Verification items for the finished model (mm, model axes). A direction names the side the tool comes from. Round coordinates to 2 decimals unless told otherwise and drop trailing zeros. Write each loop counter-clockwise with the first axis right and the second up, starting at its lowest first coordinate (ties: lowest second). Pieces come first, ordered by that corner, then holes. Notation, with made-up numbers: (-1, -39.75) - (21, -39.75) arc R22 ccw to (21, -29.75) - close; hole circle Ø7 at (-28, 8.5). An arc over 180 degrees is marked (long way). Answer as a JSON object with one key per item and string values. Group by question number.
1) Mould release check, pull along Z, two halves, no side actions. Record for faces 4 (the cylindrical face through (105.83, 3.42, 37.39)), 5 (the cylindrical face through (6.1, 8.35, 33.76)), 6 (the cylindrical face through (5.92, 3.42, -37.39)), 7 (the flat face through (0, 18, -1)): +Z half, -Z half, draft (parallel to the pull), parting line (faces both ways), or undercut.
2) Section check D-D (z = 26). State how many separate pieces and enclosed holes the cut face has, then the cut area to 3 significant figures.
3) Section check B-B (z = -16.5). Enter the section's corners in (x, y), then the cut area to 3 significant figures.
4) Set-up check for faces 1 (the flat face through (94, 53, 23)), 2 (the flat face through (69, 46, -6)), 3 (the flat face through (54, 24, -1)): record each of +Z, -Z, +X, -X, +Y, -Y from which the full face is reachable in a straight line by a thin tool's end or side.
5) Thickness scan on line 1 (Z direction, x = 7, y = 12); line 2 (Y direction, x = 106, z = 29); line 3 (Y direction, x = 5, z = -29). Record the ranges inside material, lowest first.
6) Section check A-A (x = 115). Enter the section's corners in (y, z).
7) Go/stop test with flat-tipped pins: pin 1 Ø12 at (y, z) = (16.5, 31.5) entering from -X; pin 2 Ø11 at (y, z) = (12, -29) entering from -X; pin 3 Ø12 at (y, z) = (14, 17) entering from +X; pin 4 Ø3 at (x, z) = (68, -15.5) entering from -Y. Record where each tip stops, or that it passes through.
8) Section check C-C (x = 58). Enter the section's corners in (y, z), then the cut area to 3 significant figures.
```python
from build123d import *

# Parameters (mm, degrees)
BOSS_EXTRUDE1_DEPTH              = 41
BOSS_EXTRUDE1_DEPTH_BACK         = 41
FILLET1_R                        = 12
F_12_0MM_DOWEL_HOLE1_D           = 12
F_12_0MM_DOWEL_HOLE1_CSINK_D     = 12.05
F_12_0MM_DOWEL_HOLE1_CSINK_ANGLE = 90
BOSS_EXTRUDE2_DEPTH              = 30
BOSS_EXTRUDE2_DEPTH_BACK         = 30
SKETCH8_R                        = 5
CUT_EXTRUDE1_DEPTH               = 181.113852882
BOSS_EXTRUDE3_DEPTH              = 6
BOSS_EXTRUDE3_DEPTH_BACK         = 6


with BuildPart() as part:
    # Sketch1 → Boss-Extrude1 (new, two sides: drawn at the far end of the back side and taken through both)
    with BuildSketch(Plane.XY.offset(-BOSS_EXTRUDE1_DEPTH_BACK)):
        Polygon((0, 0), (0, 36), (94, 36), (94, 70), (118, 70), (118, 0), (94, 0), (94, 24), (12, 24), (12, 0), align=None)
    extrude(amount=BOSS_EXTRUDE1_DEPTH + BOSS_EXTRUDE1_DEPTH_BACK)

    # Fillet1
    fillet1_edges = [part.edges().sort_by_distance(p)[0] for p in [
        (106, 0, -41),
        (6, 0, 41),
        (106, 0, 41),
        (6, 0, -41),
    ]]
    fillet(fillet1_edges, radius=FILLET1_R)

    # Ø12.0mm Dowel Hole1 (through all)
    with Locations(Plane.ZY):
        with Locations((-29, 12), (29, 12)):
            CounterSinkHole(F_12_0MM_DOWEL_HOLE1_D / 2, F_12_0MM_DOWEL_HOLE1_CSINK_D / 2, counter_sink_angle=F_12_0MM_DOWEL_HOLE1_CSINK_ANGLE)

    # Sketch7 → Boss-Extrude2 (add, two sides: drawn at the far end of the back side and taken through both)
    with BuildSketch(Plane.XY.offset(-BOSS_EXTRUDE2_DEPTH_BACK)):
        with BuildLine():
            Line((118, 34.22291236), (118, 70))
            Line((118, 70), (128, 70))
            Line((128, 70), (150, 70))
            ThreePointArc((150, 70), (144.397831835, 55.333333333), (130.444444444, 48.13622422))
            ThreePointArc((130.444444444, 48.13622422), (121.565016105, 43.556245693), (118, 34.22291236))
        make_face()
    extrude(amount=BOSS_EXTRUDE2_DEPTH + BOSS_EXTRUDE2_DEPTH_BACK)

    # Sketch8 → Cut-Extrude1 (cut, through all)
    with BuildSketch(Plane.XY.offset(30)):
        with Locations((128, 70)):
            Circle(SKETCH8_R)
    extrude(amount=-CUT_EXTRUDE1_DEPTH, mode=Mode.SUBTRACT)

    # Sketch9 → Boss-Extrude3 (add, two sides: drawn at the far end of the back side and taken through both)
    with BuildSketch(Plane.XY.offset(-BOSS_EXTRUDE3_DEPTH_BACK)):
        Polygon((0, 36), (94, 70), (94, 36), align=None)
    extrude(amount=BOSS_EXTRUDE3_DEPTH + BOSS_EXTRUDE3_DEPTH_BACK)


solid = part.part
```
Returned:
{
 "1": {"face 4": "+Z half", "face 5": "undercut", "face 6": "-Z half", "face 7": "draft"},
 "2": {"separate pieces": "3", "enclosed holes": "0", "area": "3,320 mm2"},
 "3": {"outline": "(0, 0) - (12, 0) - (12, 24) - (94, 24) - (94, 0) - (118, 0) - (118, 34.22) arc R14 cw to (130.44, 48.14) arc R22 ccw to (150, 70) - (133, 70) arc R5 cw to (123, 70) - (94, 70) - (94, 36) - (0, 36) - close", "area": "3,700 mm2"},
 "4": {"face 1": "+Z, -X, +Y", "face 2": "-Z, -X, +Y", "face 3": "+Z, -Z, -Y"},
 "5": {"line 1": "-41 to -35, -23 to 23, 35 to 41", "line 2": "0 to 6, 18 to 70", "line 3": "0 to 6, 18 to 36"},
 "6": {"outline": "(0, -29) arc R12 ccw to (12, -41) - (70, -41) - (70, 41) - (12, 41) arc R12 ccw to (0, 29) - close; hole circle Ø12 at (12, -29); hole circle Ø12 at (12, 29)"},
 "7": {"pin 1": "x = 0", "pin 2": "through", "pin 3": "x = 118", "pin 4": "y = 24"},
 "8": {"outline": "(24, -41) - (36, -41) - (36, -6) - (56.98, -6) - (56.98, 6) - (36, 6) - (36, 41) - (24, 41) - close", "area": "1,240 mm2"}
}
